```python
from build123d import *

# Parameters (mm, degrees)
SKETCH15_W          = 150
SKETCH15_H          = 150
SKETCH15_W_2        = 20
SKETCH15_H_2        = 5
BOSS_EXTRUDE1_DEPTH = 5


with BuildPart() as part:
    # Sketch15 → Boss-Extrude1 (new, symmetric)
    with BuildSketch(Plane(origin=(0, 0, 0), x_dir=(1, 0, 0), z_dir=(0, 1, 0))):
        Rectangle(SKETCH15_W, SKETCH15_H)
        with Locations((-25, -30.9)):
            Rectangle(SKETCH15_W_2, SKETCH15_H_2, mode=Mode.SUBTRACT)
        with Locations((25, -30.9)):
            Rectangle(SKETCH15_W_2, SKETCH15_H_2, mode=Mode.SUBTRACT)
        with Locations((25, 30.9)):
            Rectangle(SKETCH15_W_2, SKETCH15_H_2, mode=Mode.SUBTRACT)
        with Locations((-25, 30.9)):
            Rectangle(SKETCH15_W_2, SKETCH15_H_2, mode=Mode.SUBTRACT)
    extrude(amount=BOSS_EXTRUDE1_DEPTH, both=True)


with BuildPart() as part_1:
    # Body-Move/Copy1: moved
    add(part.part.moved(Location((0, -74.38, 0))))


solid = part_1.part
```
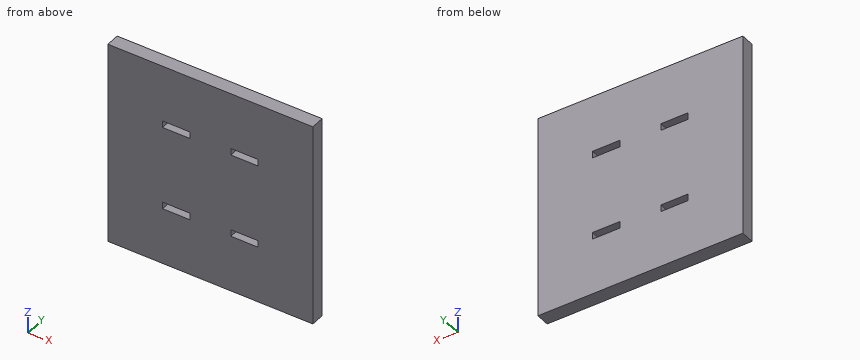
Geometry: final body of the model. Coordinates: model frame, mm. Coordinates: 2 decimals unless noted, no trailing zeros. Order: outer loops, then holes, each group sorted by start corner. A loop starts at its lowest first (then second) coordinate and runs counter-clockwise, first axis right, second up. Notation, with made-up numbers: (61.5, 0) -> (74.5, 0) arc R20 ccw to (74.5, 25) -> close; hole circle Ø4 at (24.5, 59). An arc over 180 degrees is marked (long way). Use CSV: the item, a comma, the result in double quotes.
1) Section B-B on x = 19. Output: boundary loops of the cut face in (y, z), then the cut area to 3 significant figures.
Findings:
outline,"(-79.38, -75) -> (-69.38, -75) -> (-69.38, -33.4) -> (-79.38, -33.4) -> close; (-79.38, -28.4) -> (-69.38, -28.4) -> (-69.38, 28.4) -> (-79.38, 28.4) -> close; (-79.38, 33.4) -> (-69.38, 33.4) -> (-69.38, 75) -> (-79.38, 75) -> close"
area,"1,400 mm^2"
2) Line query: line 1 (Z direction, x = 34, y = -72.5); line 2 (X direction, y = -70, z = 32). Output: solid intervals per line, ascending.
Findings:
line 1,"z = -75 to -33.4, -28.4 to 28.4, 33.4 to 75"
line 2,"x = -75 to -35, -15 to 15, 35 to 75"
3) Section A-A on y = -75. Output: boundary loops of the cut face in (x, z).
Findings:
outline,"(-75, -75) -> (75, -75) -> (75, 75) -> (-75, 75) -> close; hole (-35, -33.4) -> (-15, -33.4) -> (-15, -28.4) -> (-35, -28.4) -> close; hole (-35, 28.4) -> (-15, 28.4) -> (-15, 33.4) -> (-35, 33.4) -> close; hole (15, -33.4) -> (35, -33.4) -> (35, -28.4) -> (15, -28.4) -> close; hole (15, 28.4) -> (35, 28.4) -> (35, 33.4) -> (15, 33.4) -> close"
